Input: dimensioned drawing with shaded views. Units: mm. Origin: part minimum x, y, z. Coordinates: 2 decimals unless noted, no trailing zeros. Write each loop counter-clockwise with the first axis right and the second up, starting at its lowest first coordinate (ties: lowest second). Pieces come first, ordered by that corner, then holes. Notation, with made-up numbers: M 65.5,44.25 L 104.5,44.25 A13 cw 104.5,65.25 Z; hole C 16.5,-26.75 d5. An arc over 180 degrees is marked long. Use one line per item in the form item = value.
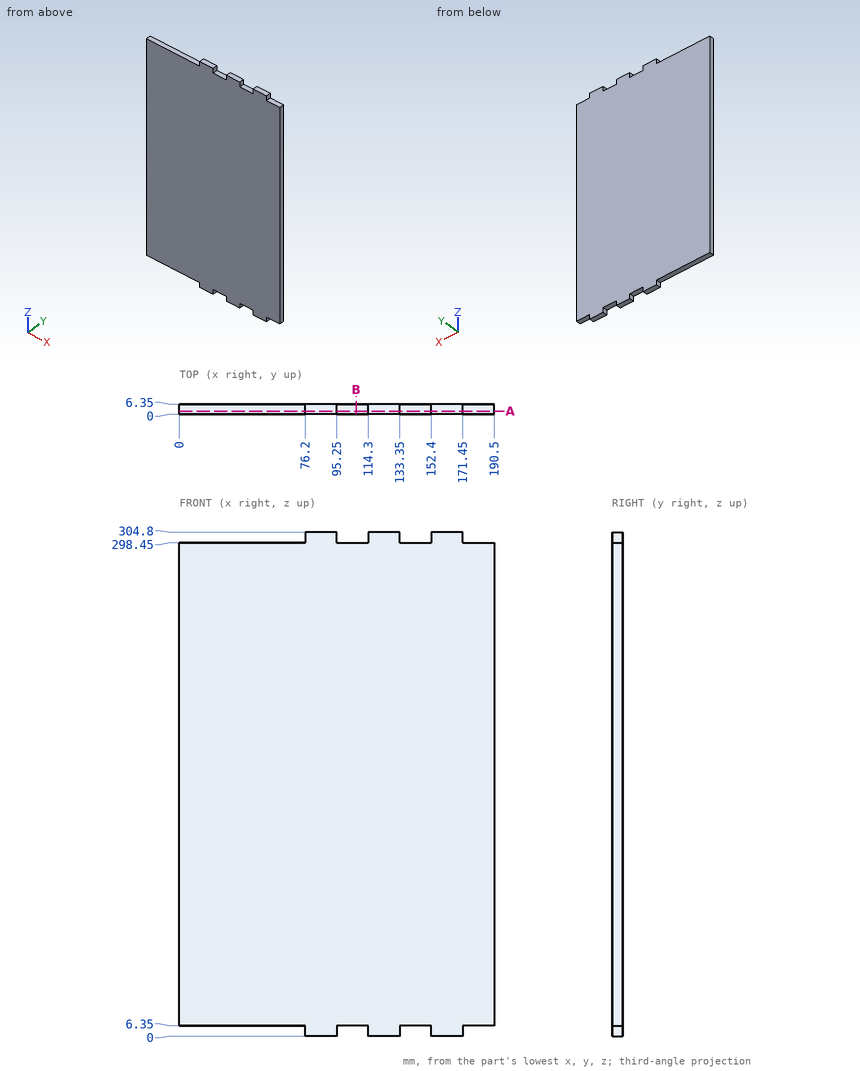
(1) Section query B-B on x = 107. Return the cut outline in (y, z), plus the area to 3 significant figures.
Computed:
outline = M 0,6.35 L 6.35,6.35 L 6.35,298.45 L 0,298.45 Z
area = 1,850 mm^2
(2) Section query A-A on y = 2. Return the cut outline in (x, z).
Computed:
outline = M 0,6.35 L 76.2,6.35 L 76.2,0 L 95.25,0 L 95.25,6.35 L 114.3,6.35 L 114.3,0 L 133.35,0 L 133.35,6.35 L 152.4,6.35 L 152.4,0 L 171.45,0 L 171.45,6.35 L 190.5,6.35 L 190.5,298.45 L 171.45,298.45 L 171.45,304.8 L 152.4,304.8 L 152.4,298.45 L 133.35,298.45 L 133.35,304.8 L 114.3,304.8 L 114.3,298.45 L 95.25,298.45 L 95.25,304.8 L 76.2,304.8 L 76.2,298.45 L 0,298.45 Z
(3) Line query: probe 1 along Z at (x, y) = (54, 2). Output: solid intervals per line, ascending.
Computed:
probe_1 = 6.35 to 298.45
(4) First-contact query: pin 1 Ø1.9 at (x, y) = (183, 4.5) entering from -Z; pin 2 Ø3 at (y, z) = (4, 3) entering from +X; pin 3 Ø1.9 at (y, z) = (3, 300.5) entering from -X. Flat tips, straight axial feed; report the tip coordinate or a pass-through.
Computed:
pin_1 = 6.35
pin_2 = 171.45
pin_3 = 76.2
